The figure shows three views and two pictorial views of one solid part (mm, origin at its lowest corner). Answer the questions. Coordinates: 2 decimals unless noted, no trailing zeros. Order: outer loops, then holes, each group sorted by start corner. A loop starts at its lowest first (then second) coordinate and runs counter-clockwise, first axis right, second up. Notation, with made-up numbers: (76.5, -1) -> (135.5, -1) arc R17 ccw to (135.5, 26) -> close; hole circle Ø11 at (54, 5). An arc over 180 degrees is marked (long way). Return JSON: item names as keys, results as strings.
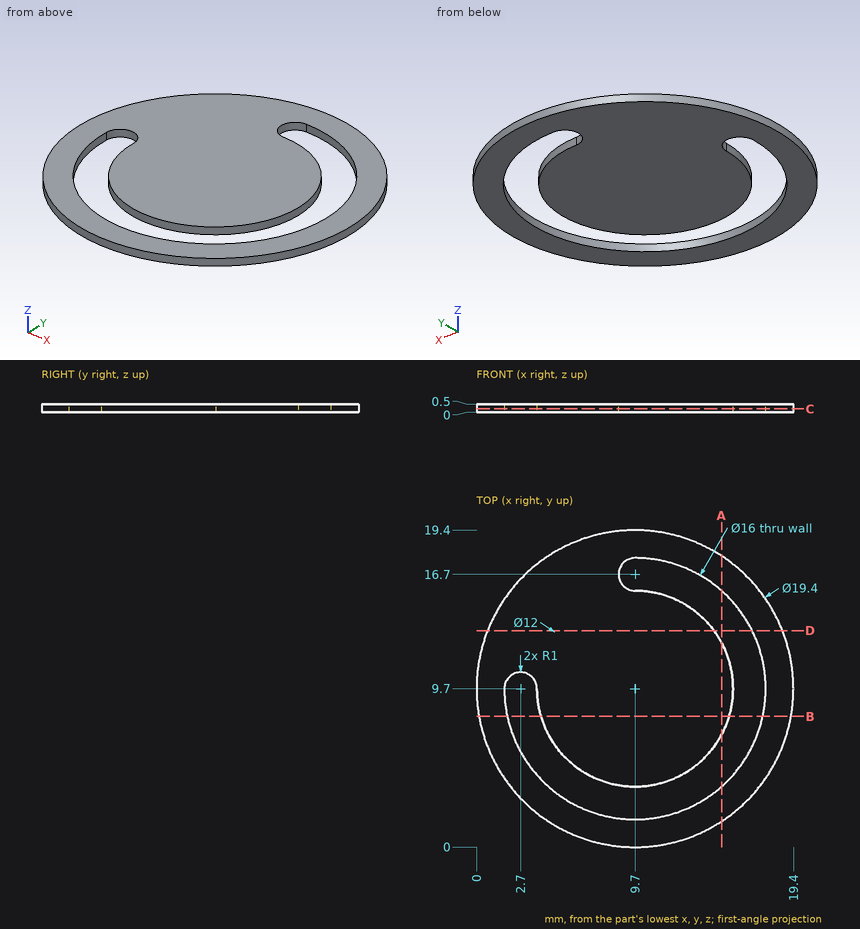
1. The part is cut by section C-C on z = 0.2. Give the vertices of the cut face in (x, y), and give its area (3 significant figures).
Answer block:
{"outline": "circle Ø19.4 at (9.7, 9.7); hole (1.7, 9.7) arc R8 ccw (long way) to (9.7, 17.7) arc R1 ccw to (9.7, 15.7) arc R6 cw (long way) to (3.7, 9.7) arc R1 ccw to start", "area": "226 mm2"}
2. The part is cut by section A-A on x = 15. Give the vertices of the cut face in (y, z).
Answer block:
{"outline": "(1.58, 0) -> (3.71, 0) -> (3.71, 0.5) -> (1.58, 0.5) -> close; (6.89, 0) -> (12.51, 0) -> (12.51, 0.5) -> (6.89, 0.5) -> close; (15.69, 0) -> (17.82, 0) -> (17.82, 0.5) -> (15.69, 0.5) -> close"}
3. The part is cut by section D-D on y = 13.25. Give the vertices of the cut face in (x, z).
Answer block:
{"outline": "(0.67, 0) -> (14.54, 0) -> (14.54, 0.5) -> (0.67, 0.5) -> close; (16.87, 0) -> (18.73, 0) -> (18.73, 0.5) -> (16.87, 0.5) -> close"}
4. This flat-tipped pin is pushed along its axis until it touches: pin 1 Ø8 at (x, y) = (11, 11.5) entering from -Z. Where does it stop, or does it pass through?
Answer block:
{"pin 1": "stops at z = 0"}
5. The part is cut by section B-B on y = 8. Give the vertices of the cut face in (x, z).
Answer block:
{"outline": "(0.15, 0) -> (1.88, 0) -> (1.88, 0.5) -> (0.15, 0.5) -> close; (3.95, 0) -> (15.45, 0) -> (15.45, 0.5) -> (3.95, 0.5) -> close; (17.52, 0) -> (19.25, 0) -> (19.25, 0.5) -> (17.52, 0.5) -> close"}
6. Consider line 1 (Y direction, x = 13.25, z = 0.2); line 2 (Y direction, x = 13.5, z = 0.25); line 3 (Y direction, x = 2.5, z = 0.4). Determine where each line is inside the solid, lowest interval first. Write a range as from..to.
Answer block:
{"line 1": "y = 0.67..2.53, 4.86..14.54, 16.87..18.73", "line 2": "y = 0.78..2.66, 5.06..14.34, 16.74..18.62", "line 3": "y = 3.2..6.21, 10.68..16.2"}
